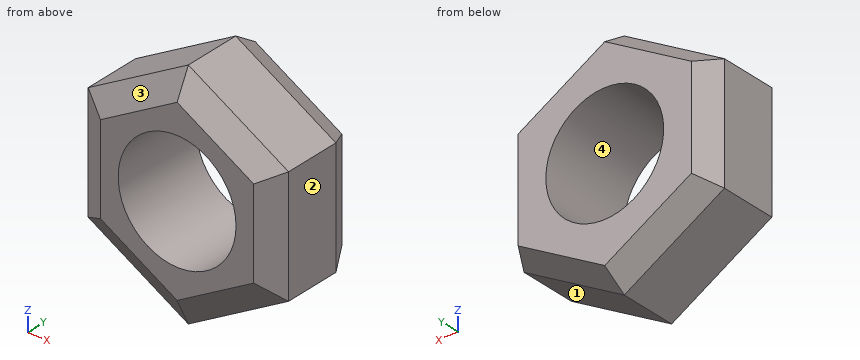
from build123d import *

# Parameters (mm, degrees)
SKETCH_1_R             = 5
EXTRUDE_1_DEPTH        = 8
CHAMFER_1_SIZE         = 2
CHAMFER_1_SIZE2        = 1.154700538
CHAMFER_1_PART_2_SIZE  = 2
CHAMFER_1_PART_2_SIZE2 = 1.154700538
CHAMFER_1_PART_3_SIZE  = 2
CHAMFER_1_PART_3_SIZE2 = 1.154700538
CHAMFER_1_PART_4_SIZE  = 2
CHAMFER_1_PART_4_SIZE2 = 1.154700538
CHAMFER_1_PART_5_SIZE  = 2
CHAMFER_1_PART_5_SIZE2 = 1.154700538
CHAMFER_1_PART_6_SIZE  = 2
CHAMFER_1_PART_6_SIZE2 = 1.154700538
CHAMFER_1_PART_7_SIZE  = 2
CHAMFER_1_PART_7_SIZE2 = 1.154700538


with BuildPart() as part:
    # Эскиз1 → Бобышка-Вытянуть1 (new body)
    with BuildSketch(Plane(origin=(0, 0, 0), x_dir=(1, 0, 0), z_dir=(0, 1, 0))):
        Polygon((8.5, -4.907477288), (8.5, 4.907477288), (0, 9.814954576), (-8.5, 4.907477288), (-8.5, -4.907477288), (0, -9.814954576), align=None)
        Circle(SKETCH_1_R, mode=Mode.SUBTRACT)
    extrude(amount=EXTRUDE_1_DEPTH)

    # Фаска1
    chamfer_1_edges = [part.edges().sort_by_distance(p)[0] for p in [
        (4.25, 8, -7.361215932),
    ]]
    chamfer_1_side = [part.faces().sort_by_distance(p)[0] for p in [
        (4.25, 4, -7.361215932),
    ]]
    chamfer(chamfer_1_edges, length=CHAMFER_1_SIZE, length2=CHAMFER_1_SIZE2, reference=chamfer_1_side[0])

    # Фаска1 part 2
    chamfer_1_part_2_edges = [part.edges().sort_by_distance(p)[0] for p in [
        (-4.25, 8, -7.361215932),
    ]]
    chamfer_1_part_2_side = [part.faces().sort_by_distance(p)[0] for p in [
        (-4.25, 4, -7.361215932),
    ]]
    chamfer(chamfer_1_part_2_edges, length=CHAMFER_1_PART_2_SIZE, length2=CHAMFER_1_PART_2_SIZE2, reference=chamfer_1_part_2_side[0])

    # Фаска1 part 3
    chamfer_1_part_3_edges = [part.edges().sort_by_distance(p)[0] for p in [
        (-8.5, 8, 0),
    ]]
    chamfer_1_part_3_side = [part.faces().sort_by_distance(p)[0] for p in [
        (-8.5, 4, 0),
    ]]
    chamfer(chamfer_1_part_3_edges, length=CHAMFER_1_PART_3_SIZE, length2=CHAMFER_1_PART_3_SIZE2, reference=chamfer_1_part_3_side[0])

    # Фаска1 part 4
    chamfer_1_part_4_edges = [part.edges().sort_by_distance(p)[0] for p in [
        (-4.25, 8, 7.361215932),
    ]]
    chamfer_1_part_4_side = [part.faces().sort_by_distance(p)[0] for p in [
        (-4.25, 4, 7.361215932),
    ]]
    chamfer(chamfer_1_part_4_edges, length=CHAMFER_1_PART_4_SIZE, length2=CHAMFER_1_PART_4_SIZE2, reference=chamfer_1_part_4_side[0])

    # Фаска1 part 5
    chamfer_1_part_5_edges = [part.edges().sort_by_distance(p)[0] for p in [
        (4.25, 8, 7.361215932),
    ]]
    chamfer_1_part_5_side = [part.faces().sort_by_distance(p)[0] for p in [
        (4.25, 4, 7.361215932),
    ]]
    chamfer(chamfer_1_part_5_edges, length=CHAMFER_1_PART_5_SIZE, length2=CHAMFER_1_PART_5_SIZE2, reference=chamfer_1_part_5_side[0])

    # Фаска1 part 6
    chamfer_1_part_6_edges = [part.edges().sort_by_distance(p)[0] for p in [
        (-4.25, 0, 7.361215932),
        (-8.5, 0, 0),
        (-4.25, 0, -7.361215932),
        (4.25, 0, -7.361215932),
        (8.5, 0, 0),
        (4.25, 0, 7.361215932),
    ]]
    chamfer_1_part_6_side = [part.faces().sort_by_distance(p)[0] for p in [
        (8.240320711, 0, 0),
    ]]
    chamfer(chamfer_1_part_6_edges, length=CHAMFER_1_PART_6_SIZE, length2=CHAMFER_1_PART_6_SIZE2, reference=chamfer_1_part_6_side[0])

    # Фаска1 part 7
    chamfer_1_part_7_edges = [part.edges().sort_by_distance(p)[0] for p in [
        (8.5, 8, 0),
    ]]
    chamfer_1_part_7_side = [part.faces().sort_by_distance(p)[0] for p in [
        (8.5, 4, 0),
    ]]
    chamfer(chamfer_1_part_7_edges, length=CHAMFER_1_PART_7_SIZE, length2=CHAMFER_1_PART_7_SIZE2, reference=chamfer_1_part_7_side[0])


solid = part.part
Work out the finished part from the listing and answer in its coordinate system (mm). Face numbers are marked on the shaded views. Give positions to 0.01 mm unless a question says otherwise; leave off trailing zeros. Loops run counter-clockwise (first coordinate to the right, second up) from the corner with the lowest first, then second, coordinate; pieces in that order, holes last. Notation, with made-up numbers: (45, -36) -> (95, -36) arc R28 ccw to (95, -18) -> close; hole circle Ø2 at (73, 25.5). An arc over 180 degrees is marked (long way). Use a Markdown table: item, result. Add a question column.
1) The part is cut by section C-C, the plane x = -1.5. Determine the outline of the cut face in (y, z).
2) The part is cut by section A-A, the plane y = 2.25. Determine the outline of the cut face in (x, z).
3) For a pull along Z with two mould halves and no side action, classify the marked faces 1, 2, 3 and 4 as +Z half, -Z half, draft (parallel to the pull), parting line (faces both ways), or undercut.
4) Consider line 1 along X through (y, z) = (2.75, 0); line 2 along Z through (x, y) = (-2, 3.5); line 3 along X through (y, z) = (3, 2.25). Determine where each line is inside the solid, lowest interval first.
5) The part is cut by section B-B, the plane z = 0. Determine the outline of the cut face in (x, y).
6) Each of these flat-tipped pins is pushed along its axis until it touches: P1, Ø1.5, axis at y = 3, z = -6, coming from the +X side; P2, Ø2, axis at x = 3.5, z = -7, coming from the +Y side; P3, Ø1, axis at x = -2, y = 3.5, coming from the +Z side; P4, Ø3, axis at x = -5, y = 5.5, coming from the -Z side. Where does it stop, or does it pass through?
7) The part is cut by section D-D, the plane z = -5.5. Determine the outline of the cut face in (x, y), plus the area to 3 significant figures.
Reported:
| question | item | result |
|---|---|---|
| 1 | outline | (0, -6.64) -> (1.15, -8.95) -> (6, -8.95) -> (8, -7.62) -> (8, -4.77) -> (0, -4.77) -> close; (0, 4.77) -> (8, 4.77) -> (8, 7.62) -> (6, 8.95) -> (1.15, 8.95) -> (0, 6.64) -> close |
| 2 | outline | (-8.5, -4.91) -> (0, -9.81) -> (8.5, -4.91) -> (8.5, 4.91) -> (0, 9.81) -> (-8.5, 4.91) -> close; hole circle Ø10 at (0, 0) |
| 3 | face 1 | -Z half |
| 3 | face 2 | draft |
| 3 | face 3 | +Z half |
| 3 | face 4 | undercut |
| 4 | line 1 | x = -8.5 to -5, 5 to 8.5 |
| 4 | line 2 | z = -8.66 to -4.58, 4.58 to 8.66 |
| 4 | line 3 | x = -8.5 to -4.47, 4.47 to 8.5 |
| 5 | outline | (-8.5, 1.15) -> (-6.5, 0) -> (-5, 0) -> (-5, 8) -> (-7.35, 8) -> (-8.5, 6) -> close; (5, 0) -> (6.5, 0) -> (8.5, 1.15) -> (8.5, 6) -> (7.35, 8) -> (5, 8) -> close |
| 6 | P1 | stops at x = 7.91 |
| 6 | P2 | stops at y = 8 |
| 6 | P3 | stops at z = 8.95 |
| 6 | P4 | stops at z = -7.79 |
| 7 | outline | (-7.47, 1.15) -> (-3.47, 0) -> (3.47, 0) -> (7.47, 1.15) -> (7.47, 6) -> (5.16, 8) -> (-5.16, 8) -> (-7.47, 6) -> close |
| 7 | area | 110 mm^2 |
